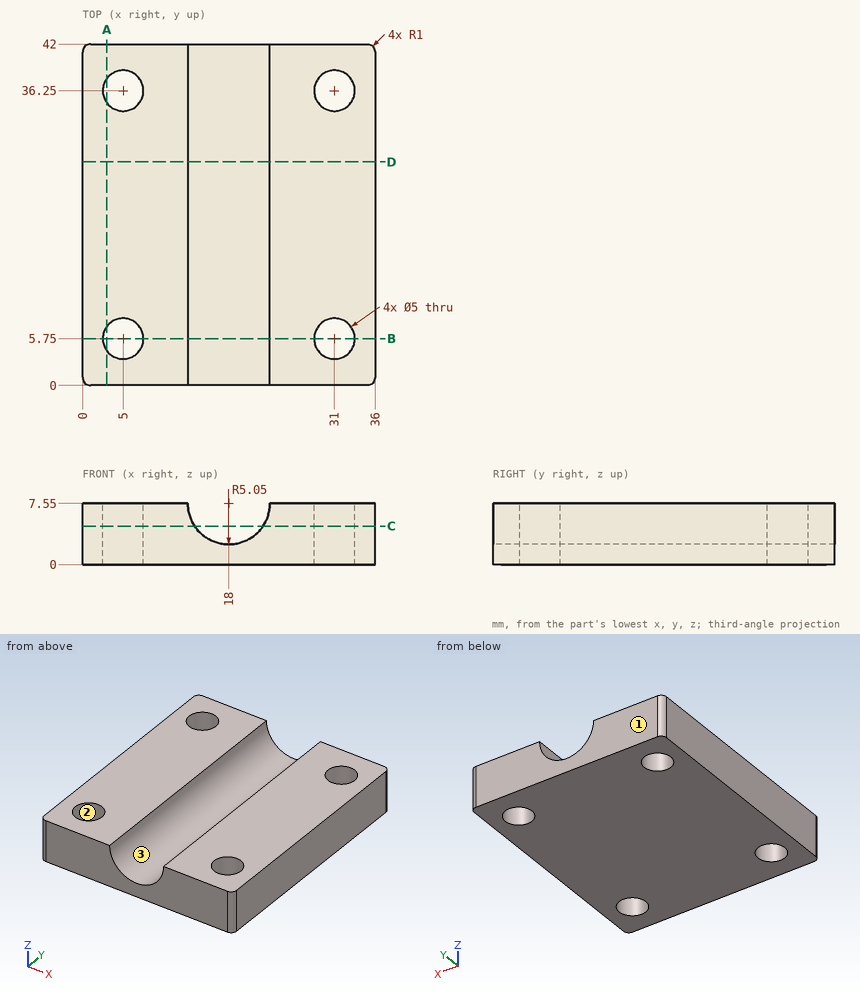
Here's the drawing with two shaded views (mm, measured from the low corner). I have some questions. Coordinates: 2 decimals unless noted, no trailing zeros. Loops run counter-clockwise (first coordinate to the right, second up) from the corner with the lowest first, then second, coordinate; pieces in that order, holes last. Notation, with made-up numbers: M 69.5,1.25 L 113.5,1.25 A15 ccw 113.5,24.25 Z; hole C -37.5,85.5 d5. An arc over 180 degrees is marked long. Return JSON: item names as keys, results as strings. Group by question number.
Item 1: Imagine slicing it at A-A (x = 3). Please give me the cut outline in (y, z).
Item 2: I'm going to push flat-ended pins straight in: pin 1 Ø4.5 at (x, y) = (31, 36.25) entering from +Z; pin 2 Ø1.5 at (x, y) = (21.5, 33.5) entering from -Z. Where does each tip first touch, or does it pass through?
Item 3: Imagine slicing it at B-B (y = 5.75). Please give me the cut outline in (x, z).
Item 4: Thinking about a two-plate mould opening in Y: for the marked faces 1, 2 and 3, which applies, released by +Y, released by -Y, zero draft, split by the parting line, or undercut?
Item 5: If I drill on L1, parallel to Y at x = 31, z = 4; L2, parallel to X at y = 36.5, z = 3.25; L3, parallel to X at y = 5.75, z = 3, over which ranges is the centre line in solid material (lowest first)? Write a range as from..to.
Item 6: Imagine slicing it at C-C (z = 4.75). Please give me the cut outline in (x, y).
Item 7: Imagine slicing it at D-D (y = 27.5). Please give me the cut outline in (x, z), and give its area (3 significant figures).
Verdict:
{
 "1": {"outline": "M 0,0 L 4.25,0 L 4.25,7.55 L 0,7.55 Z; M 7.25,0 L 34.75,0 L 34.75,7.55 L 7.25,7.55 Z; M 37.75,0 L 42,0 L 42,7.55 L 37.75,7.55 Z"},
 "2": {"pin 1": "passes through", "pin 2": "stops at z = 0"},
 "3": {"outline": "M 0,0 L 2.5,0 L 2.5,7.55 L 0,7.55 Z; M 7.5,0 L 28.5,0 L 28.5,7.55 L 23.05,7.55 A5.05 cw 12.95,7.55 L 7.5,7.55 Z; M 33.5,0 L 36,0 L 36,7.55 L 33.5,7.55 Z"},
 "4": {"face 1": "released by +Y", "face 2": "undercut", "face 3": "zero draft"},
 "5": {"L1": "y = 0..3.25, 8.25..33.75, 38.75..42", "L2": "x = 0..2.51, 7.49..15.35, 20.65..28.51, 33.49..36", "L3": "x = 0..2.5, 7.5..15.81, 20.19..28.5, 33.5..36"},
 "6": {"outline": "M 0,1 A1 ccw 1,0 L 13.8,0 L 13.8,42 L 1,42 A1 ccw 0,41 Z; M 22.2,0 L 35,0 A1 ccw 36,1 L 36,41 A1 ccw 35,42 L 22.2,42 Z; hole C 5,5.75 d5; hole C 5,36.25 d5; hole C 31,5.75 d5; hole C 31,36.25 d5"},
 "7": {"outline": "M 0,0 L 36,0 L 36,7.55 L 23.05,7.55 A5.05 cw 12.95,7.55 L 0,7.55 Z", "area": "232 mm^2"}
}
